Geometry: final body of the model. Coordinates: model frame, mm. Face numbers are marked on the shaded views. A direction names the side the tool comes from. Coordinates: 2 decimals unless noted, no trailing zeros. Loops run counter-clockwise (first coordinate to the right, second up) from the corner with the lowest first, then second, coordinate; pieces in that order, holes last. Notation, with made-up numbers: (-15.75, -29.75) - (36.25, -29.75) arc R19 cw to (36.25, -12.75) - close; hole circle Ø5 at (76, 78). An arc over 180 degrees is marked (long way). Return JSON: item names as keys, results as strings.
from build123d import *

# Parameters (mm, degrees)
BODY_DEPTH         = 65
CUT_EXTRUDE1_DEPTH = 3
SKETCH5_R          = 19
SKETCH5_R_2        = 2.6
CUT_EXTRUDE2_DEPTH = 3


with BuildPart() as part:
    # Sketch1 → Body (new body)
    with BuildSketch(Plane(origin=(0, 0, 0), x_dir=(0, 0, -1), z_dir=(1, 0, 0))):
        with BuildLine():
            Line((0, 0), (-66, 0))
            ThreePointArc((-66, 0), (-67.414213562, 0.585786438), (-68, 2))
            Line((-68, 2), (-68, 80.25))
            Line((-68, 80.25), (-65, 80.25))
            Line((-65, 80.25), (-65, 5))
            ThreePointArc((-65, 5), (-64.414213562, 3.585786438), (-63, 3))
            Line((-63, 3), (0, 3))
            Line((0, 3), (0, 0))
        make_face()
    extrude(amount=BODY_DEPTH)

    # Sketch4 → Cut-Extrude1 (cut)
    with BuildSketch(Plane(origin=(0, 3, 0), x_dir=(1, 0, 0), z_dir=(0, 1, 0))):
        with BuildLine():
            Line((50.4, -52), (50.4, -10))
            ThreePointArc((50.4, -10), (52.5, -7.9), (54.6, -10))
            Line((54.6, -10), (54.6, -52))
            ThreePointArc((54.6, -52), (52.5, -54.1), (50.4, -52))
        make_face()
        with BuildLine():
            Line((10.4, -52), (10.4, -10))
            ThreePointArc((10.4, -10), (12.5, -7.9), (14.6, -10))
            Line((14.6, -10), (14.6, -52))
            ThreePointArc((14.6, -52), (12.5, -54.1), (10.4, -52))
        make_face()
    extrude(amount=-CUT_EXTRUDE1_DEPTH, mode=Mode.SUBTRACT)

    # Sketch5 → Cut-Extrude2 (cut)
    with BuildSketch(Plane(origin=(0, 0, 65), x_dir=(-1, 0, 0), z_dir=(0, 0, -1))):
        with Locations((-32.5, 51.25)):
            Circle(SKETCH5_R)
        with Locations((-9, 74.75)):
            Circle(SKETCH5_R_2)
        with Locations((-56, 74.75)):
            Circle(SKETCH5_R_2)
        with Locations((-56, 27.75)):
            Circle(SKETCH5_R_2)
        with Locations((-9, 27.75)):
            Circle(SKETCH5_R_2)
    extrude(amount=-CUT_EXTRUDE2_DEPTH, mode=Mode.SUBTRACT)


solid = part.part
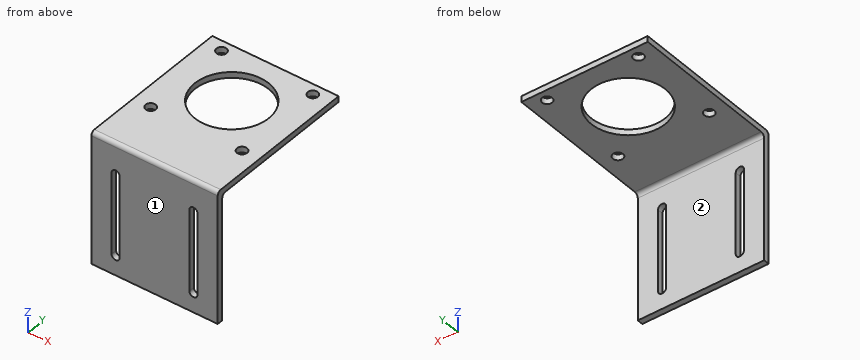
Item 1: Reachability of the marked faces 1 and 2 from +Z, -Z, +X, -X, +Y, -Y: full face, straight path, thin tool, end or side. Return the list, or none.
Worked out:
{"face 1": "+Z, -Z, +X, -X, -Y", "face 2": "-Z, +X, -X, +Y"}
Item 2: Section query B-B, the plane z = 19. Return loops of the section in (x, y), and give its area (3 significant figures).
Worked out:
{"outline": "(0, 0) - (10.4, 0) - (10.4, 3) - (0, 3) - close; (14.6, 0) - (50.4, 0) - (50.4, 3) - (14.6, 3) - close; (54.6, 0) - (65, 0) - (65, 3) - (54.6, 3) - close", "area": "170 mm^2"}
Item 3: Section query C-C, the plane y = 27.75. Return loops of the section in (x, z), and give its area (3 significant figures).
Worked out:
{"outline": "(0, 65) - (6.4, 65) - (6.4, 68) - (0, 68) - close; (11.6, 65) - (53.4, 65) - (53.4, 68) - (11.6, 68) - close; (58.6, 65) - (65, 65) - (65, 68) - (58.6, 68) - close", "area": "164 mm^2"}
Item 4: Ray query, probe 1 along Y at (x, z) = (9, 66); probe 2 along X at (y, z) = (51, 66); probe 3 along Y at (x, z) = (32.5, 66). Return the intervals inside material, ascending. Write a range as from..to.
Worked out:
{"probe 1": "0..25.15, 30.35..72.15, 77.35..80.25", "probe 2": "0..13.5, 51.5..65", "probe 3": "0..32.25, 70.25..80.25"}
Item 5: First-contact query: pin 1 Ø6 at (x, y) = (30, 65.5) entering from +Z; pin 2 Ø19.5 at (x, y) = (31, 33.5) entering from -Z; pin 3 Ø1 at (x, z) = (6.5, 26.5) entering from +Y. Flat tips, straight axial feed; report the tip coordinate or a pass-through.
Worked out:
{"pin 1": "through", "pin 2": "z = 65", "pin 3": "y = 3"}
Item 6: Section query D-D, the plane y = 51.25. Return loops of the section in (x, z).
Worked out:
{"outline": "(0, 65) - (13.5, 65) - (13.5, 68) - (0, 68) - close; (51.5, 65) - (65, 65) - (65, 68) - (51.5, 68) - close"}
Item 7: Section query A-A, the plane x = 56. Return loops of the section in (y, z), and give its area (3 significant figures).
Worked out:
{"outline": "(0, 0) - (3, 0) - (3, 63) arc R2 cw to (5, 65) - (25.15, 65) - (25.15, 68) - (2, 68) arc R2 ccw to (0, 66) - close; (30.35, 65) - (72.15, 65) - (72.15, 68) - (30.35, 68) - close; (77.35, 65) - (80.25, 65) - (80.25, 68) - (77.35, 68) - close", "area": "405 mm^2"}
